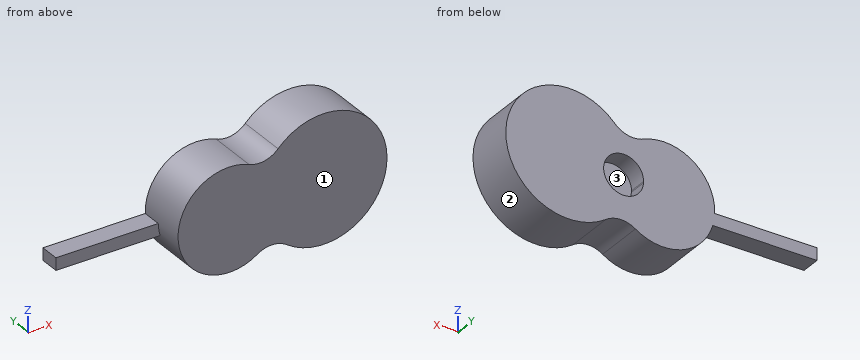
from build123d import *

# Parameters (mm, degrees)
F1_DEPTH = 9.652
F2_W     = 22.6732008159
F2_H     = 1.1748634279
F2_H_2   = 1.2006908655
F3_DEPTH = 3.81
F4_R     = 5.08
F6_DEPTH = 3.556


with BuildPart() as f1:
    # F0 (on Front) → F1 (new body)
    with BuildSketch(Plane.XZ):
        with BuildLine():
            ThreePointArc((-31.5301379097, 29.2723811601), (-9.2584932634, 37.5565839315), (-32.6741015598, 41.6017611729))
            ThreePointArc((-32.6741015598, 41.6017611729), (-49.691111152, 33.8051020972), (-31.5301379097, 29.2723811601))
        make_face()
    extrude(amount=F1_DEPTH)

    # F2 (on Front) → F3 (join)
    with BuildSketch(Plane.XZ):
        with Locations((-58.2245606929, 33.776761964)):
            Rectangle(F2_W, F2_H)
        with Locations((-58.2245606929, 32.5889848173)):
            Rectangle(F2_W, F2_H_2)
    extrude(amount=F3_DEPTH)

    # F4
    f4_edges = [f1.edges().sort_by_distance(p)[0] for p in [
        (-32.674102, -4.826, 41.601761),
        (-31.530138, -4.826, 29.272381),
    ]]
    fillet(f4_edges, radius=F4_R)

    # F5 (on face) → F6 (cut)
    with BuildSketch(Plane(origin=(0, 0, 0), x_dir=(-1, 0, 0), z_dir=(0, 1, 0))):
        with BuildLine():
            ThreePointArc((35.9255568085, 35.9008908942), (32.1931363304, 39.7711420697), (28.1901409202, 36.1814576083))
            Line((28.1901409202, 36.1814576083), (35.9153805385, 35.6203241801))
            ThreePointArc((35.9153805385, 35.6203241801), (35.9230119048, 35.7605152931), (35.9255568085, 35.9008908942))
        make_face()
        with BuildLine():
            Line((35.9153805385, 35.6203241801), (28.1901409202, 36.1814576083))
            ThreePointArc((28.1901409202, 36.1814576083), (31.7721940152, 32.038271085), (35.9153805385, 35.6203241801))
        make_face()
    extrude(amount=-F6_DEPTH, mode=Mode.SUBTRACT)


solid = f1.part
Geometry check sheet. Reference: the model listing, model coordinates, mm. Face numbers are marked on the shaded views. Round coordinates to 2 decimals unless told otherwise and drop trailing zeros. Order: outer loops, then holes, each group sorted by start corner. A loop starts at its lowest first (then second) coordinate and runs counter-clockwise, first axis right, second up. Notation, with made-up numbers: (42, 41.25) -> (61, 41.25) arc R18 ccw to (61, 47.25) -> close; hole circle Ø10 at (50, 34.25). An arc over 180 degrees is marked (long way). Use one line per item in the form item = value.
1. Cross-section at C-C, the plane z = 28.75. Enter the section's corners in (x, y), plus the area to 3 significant figures.
Working result:
outline = (-47.73, -9.65) -> (-11.89, -9.65) -> (-11.89, 0) -> (-47.73, 0) -> close
area = 346 mm^2
2. Scan lines: line 1 along Z through (x, y) = (-21, -5); line 2 along X through (y, z) = (-3, 36.25) (3 decimals); line 3 along X through (y, z) = (-0.25, 36.75). Record each from-to range of solid material in increasing order. Write a range as from..to.
Working result:
line_1 = 24.12..48.72
line_2 = -49.615..-35.91, -28.196..-9.207
line_3 = -49.52..-35.83, -28.27..-9.21
3. Cross-section at A-A, the plane z = 32.75. Enter the section's corners in (x, y).
Working result:
outline = (-69.56, -3.81) -> (-49.54, -3.81) -> (-49.54, -9.65) -> (-9.77, -9.65) -> (-9.77, 0) -> (-29.8, 0) -> (-29.8, -3.56) -> (-34.3, -3.56) -> (-34.3, 0) -> (-69.56, 0) -> close
4. Cross-section at B-B, the plane x = -62. Enter the section's corners in (y, z), plus the area to 3 significant figures.
Working result:
outline = (-3.81, 31.99) -> (0, 31.99) -> (0, 34.36) -> (-3.81, 34.36) -> close
area = 9.05 mm^2
5. Go/stop test with flat-tipped pins: pin 1 (1.5 mm diameter, centred on x = -44.5, z = 46, fed in from +Y); pin 2 (1 mm diameter, centred on y = -6.5, z = 45.5, fed in from +X); pin 3 (12 mm diameter, centred on x = -50.5, z = 41, fed in from +Y); pin 4 (4 mm diameter, centred on x = -32, z = 35.5, fed in from +Y). Record where each tip stops, or that it passes through.
Working result:
pin_1 = through
pin_2 = -12.69
pin_3 = 0
pin_4 = -3.56
6. Mould release check, pull along Z, two halves, no side actions. Record for the marked faces 1, 2 and 3: pulls with the +Z half, pulls with the -Z half, needs draft (parallel to the pull), parting line crosses it, or undercut.
Working result:
face_1 = needs draft
face_2 = parting line crosses it
face_3 = undercut
